```python
from build123d import *

# Parameters (mm, degrees)
F0_R     = 22.165
F0_R_2   = 0.79
F0_R_3   = 5
F0_W     = 0.864478
F0_H     = 4.103523
F1_DEPTH = 1.18
F2_R     = 5
F2_R_2   = 3.975
F3_DEPTH = 2.86
F2_R_3   = 3
F4_DEPTH = 6.14
F2_R_4   = 1.435
F5_DEPTH = 0.5
F6_SIZE  = 1
F7_DEPTH = 25


with BuildPart() as f1:
    # F0 (on Top) → F1 (new body, symmetric)
    with BuildSketch(Plane.XY):
        Circle(F0_R)
        with Locations((-13.67191, -13.67191)):
            Circle(F0_R_2, mode=Mode.SUBTRACT)
        with Locations((0, -19.335)):
            Circle(F0_R_2, mode=Mode.SUBTRACT)
        with Locations((13.67191, -13.67191)):
            Circle(F0_R_2, mode=Mode.SUBTRACT)
        with Locations((-19.335, 0)):
            Circle(F0_R_2, mode=Mode.SUBTRACT)
        with Locations((-13.67191, 13.67191)):
            Circle(F0_R_2, mode=Mode.SUBTRACT)
        Circle(F0_R_3, mode=Mode.SUBTRACT)
        with Locations((19.335, 0)):
            Circle(F0_R_2, mode=Mode.SUBTRACT)
        with Locations((0, 15.216693)):
            Rectangle(F0_W, F0_H, mode=Mode.SUBTRACT)
        with Locations((0, 19.335)):
            Circle(F0_R_2, mode=Mode.SUBTRACT)
        with Locations((13.67191, 13.67191)):
            Circle(F0_R_2, mode=Mode.SUBTRACT)
        with Locations((0, 15.216693)):
            Rectangle(F0_W, F0_H)
    extrude(amount=F1_DEPTH, both=True)

    # F2 (on face) → F3 (join)
    with BuildSketch(Plane(origin=(0, 0, -1.18), x_dir=(1, 0, 0), z_dir=(0, 0, -1))):
        Circle(F2_R)
        Circle(F2_R_2, mode=Mode.SUBTRACT)
    extrude(amount=-F3_DEPTH)

    # F2 (on face) → F4 (join)
    with BuildSketch(Plane(origin=(0, 0, -1.18), x_dir=(1, 0, 0), z_dir=(0, 0, -1))):
        Circle(F2_R_2)
        Circle(F2_R_3, mode=Mode.SUBTRACT)
    extrude(amount=-F4_DEPTH)

    # F2 (on face) → F5 (join)
    with BuildSketch(Plane(origin=(0, 0, -1.18), x_dir=(1, 0, 0), z_dir=(0, 0, -1))):
        Circle(F2_R_3)
        Circle(F2_R_4, mode=Mode.SUBTRACT)
    extrude(amount=-F5_DEPTH)

    # F6
    f6_edges = [f1.edges().sort_by_distance(p)[0] for p in [
        (-3.975, 0, 1.68),
    ]]
    chamfer(f6_edges, length=F6_SIZE)

    # F0 (on Top) → F7 (cut)
    with BuildSketch(Plane.XY):
        with Locations((0, 15.216693)):
            Rectangle(F0_W, F0_H)
    extrude(amount=-F7_DEPTH, mode=Mode.SUBTRACT)


solid = f1.part
```
The listing builds one solid part. Answer for the finished solid, in the listing's coordinates (mm). A direction names the side the tool comes from. Give positions to 0.01 mm unless a question says otherwise; leave off trailing zeros. Write each loop counter-clockwise with the first axis right and the second up, starting at its lowest first coordinate (ties: lowest second). Pieces come first, ordered by that corner, then holes. Notation, with made-up numbers: (-0.5, 24) -> (35.5, 24) arc R23 ccw to (35.5, 37) -> close; hole circle Ø9 at (-11, 4.5). An arc over 180 degrees is marked (long way). Write item = value, one per line. Start each with the question number.
1) The part is cut by section A-A, the plane y = 0. Count the separate pieces of the cut face and the enclosed holes in it, and give its area (3 significant figures).
2) Determine the mould class of faces 4 (the face through (-3, 0, 2)), 5 (the face through (-0.3, 5.2, 1.18)), 6 (the face through (14.1, -13.01, -0.02)), 7 (the face through (11.9, 18.7, 0)) for opening direction X: +X half, -X half, draft (parallel to the pull), parting line (faces both ways), or undercut.
3) The part is cut by section B-B, the plane z = 4.25. Determine the outline of the cut face in (x, y) (3 decimals).
4) The part is cut by section D-D, the plane x = 17. Determine the outline of the cut face in (y, z), and give its area (3 significant figures).
5) Each of these flat-tipped pins is pushed along its axis until it touches: pin 1 (1.5 mm diameter, centred on x = -2, z = 0.5, fed in from -Y); pin 2 (3 mm diameter, centred on x = 1, y = -0.5, fed in from +Z); pin 3 (0.7 mm diameter, centred on x = 0, z = -1, fed in from +Y) (3 decimals). Where does it stop, or does it pass through?
6) Which of the six approach directions +Z, -Z, +X, -X, +Y, -Y give full straight-line access (tool end or side, diameter ignored) to faces 1 (the face through (0.432, 15, -1)), 2 (the face through (-14.46, 13.71, -0.02)), 3 (the face through (-1.08, 4.88, 1.43))?
7) The part is cut by section C-C, the plane x = -16. Determine the outline of the cut face in (y, z).
8) Straight lines are drawn through the part: line 1 along Y through (x, z) = (0, 0.2) (3 decimals); line 2 along Z through (x, y) = (-16, -11); line 3 along X through (y, z) = (14.5, -1). For each, find the intervals that lie inside material, in ascending order.
Solutions:
q1.separate_pieces = 4
q1.enclosed_holes = 0
q1.area = 94.0 mm²
q2.face_4 = undercut
q2.face_5 = draft
q2.face_6 = undercut
q2.face_7 = parting line
q3.outline = circle Ø7.95 at (0, 0); hole circle Ø6 at (0, 0)
q4.outline = (-14.22, -1.18) -> (14.22, -1.18) -> (14.22, 1.18) -> (-14.22, 1.18) -> close
q4.area = 67.1 mm²
q5.pin_1 = -22.13
q5.pin_2 = -0.68
q5.pin_3 = 22.165
q6.face_1 = -Z
q6.face_2 = +Z, -Z
q6.face_3 = +Z
q7.outline = (-15.34, -1.18) -> (15.34, -1.18) -> (15.34, 1.18) -> (-15.34, 1.18) -> close
q8.line_1 = -22.165 to -20.125, -18.545 to -3, 3 to 18.545, 20.125 to 22.165
q8.line_2 = -1.18 to 1.18
q8.line_3 = -16.76 to -0.43, 0.43 to 16.76
